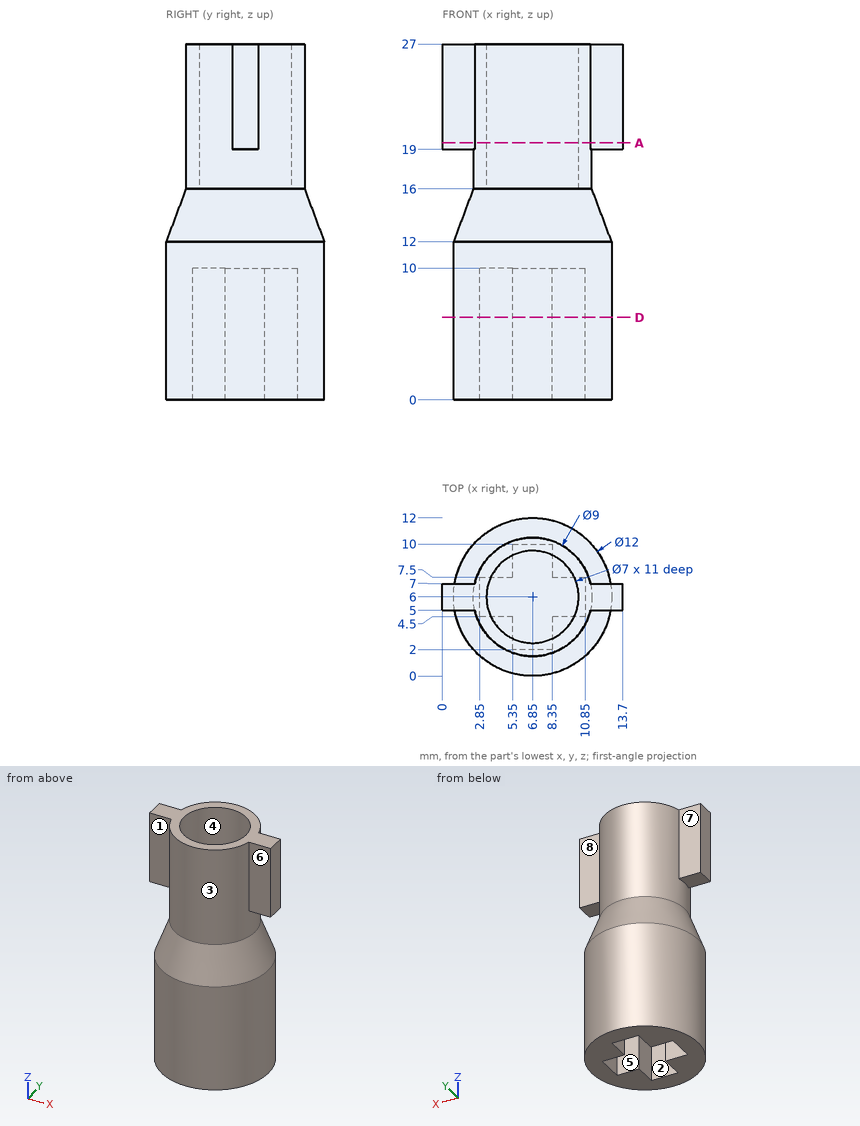
Print and shaded views of the part. All mm, measured from the part's lowest x, y and z. A direction names the side the tool comes from. Give positions to 0.01 mm unless a question says otherwise; leave off trailing zeros. Loops run counter-clockwise (first coordinate to the right, second up) from the corner with the lowest first, then second, coordinate; pieces in that order, holes last.
1) Saw through at D-D (z = 6.25). Write the cut outline in (x, y), plus the area to 3 significant figures.
2) Saw through at A-A (z = 19.5). Write the cut outline in (x, y).
3) Pull direction X, two halves, no side cores. Call the marked faces 1, 2 and 3: +X half, -X half, draft (parallel to the pull), parting line (faces both ways), or undercut.
4) Tool access for the marked faces 4, 5, 6, 7 and 8: list every direction of +Z, -Z, +X, -X, +Y, -Y with a clear straight run to the whole face (end or side of a thin tool).
5) Flat gauge pins, fed straight in: pin 1 Ø0.7 at (x, z) = (1.5, 24) entering from +Y; pin 2 Ø3.5 at (y, z) = (5.5, 6) entering from -X; pin 3 Ø1.5 at (x, z) = (11, 20.5) entering from -Y; pin 4 Ø3 at (x, y) = (10.5, 9.5) entering from +Z. Where does each tip first touch, or does it go through?
6) Wall check: line 1 (Y direction, x = 6.85, z = 18.5); line 2 (Z direction, x = 7, y = 2.75); line 3 (X direction, y = 2.25, z = 1.75). Give the ranges that are in metal, low to high.
Answer block:
1. outline: circle Ø12 at (6.85, 6); hole (2.85, 4.5) - (5.35, 4.5) - (5.35, 2) - (8.35, 2) - (8.35, 4.5) - (10.85, 4.5) - (10.85, 7.5) - (8.35, 7.5) - (8.35, 10) - (5.35, 10) - (5.35, 7.5) - (2.85, 7.5) - close
1. area: 74.1 mm2
2. outline: (0, 5) - (2.46, 5) arc R4.5 ccw to (11.24, 5) - (13.7, 5) - (13.7, 7) - (11.24, 7) arc R4.5 ccw to (2.46, 7) - (0, 7) - close; hole circle Ø7 at (6.85, 6)
3. face 1: draft
3. face 2: undercut
3. face 3: parting line
4. face 4: +Z
4. face 5: -Z
4. face 6: +Z, +X, -Y
4. face 7: +Z, -X, +Y
4. face 8: +Z, +X, +Y
5. pin 1: stops at y = 7
5. pin 2: stops at x = 0.85
5. pin 3: stops at y = 3.05
5. pin 4: stops at z = 27
6. line 1: y = 1.5 to 2.5, 9.5 to 10.5
6. line 2: z = 10 to 16
6. line 3: x = 2.17 to 5.35, 8.35 to 11.53
